from build123d import *

# Parameters (mm, degrees)
SKICA1_R                 = 60
VYSUNOUT1_DEPTH          = 10
SKICA7_R                 = 7.5
ODEBRAT_VYSUNUT_M1_DEPTH = 11
KRUHOV_POLE1_COUNT       = 6


with BuildPart() as part:
    # Skica1 → Vysunout1 (new body)
    with BuildSketch(Plane.XY):
        Circle(SKICA1_R)
    extrude(amount=VYSUNOUT1_DEPTH)

    # Skica7 → Odebrat vysunutím1 (cut, through all)
    with BuildSketch(Plane(origin=(0, 0, 0), x_dir=(-1, 0, 0), z_dir=(0, 0, -1))):
        with Locations((0, 40)):
            Circle(SKICA7_R)
    odebrat_vysunut_m1 = extrude(amount=-ODEBRAT_VYSUNUT_M1_DEPTH, mode=Mode.SUBTRACT)

    # Kruhové pole1: Odebrat vysunutím1 ×6 about axis
    kruhov_pole1_axis = Axis((0, 0, 0), (0, 0, 1))
    for i in range(1, KRUHOV_POLE1_COUNT):
        add(odebrat_vysunut_m1.rotate(kruhov_pole1_axis, i * 360 / KRUHOV_POLE1_COUNT), mode=Mode.SUBTRACT)


solid = part.part
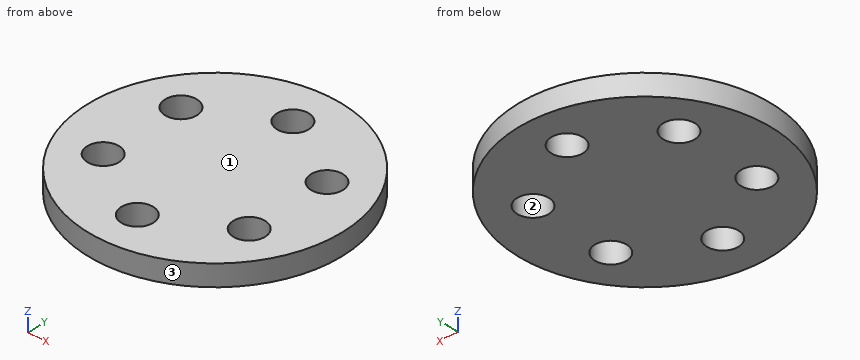
Part model, mm, in its own coordinate system. Face numbers are marked on the shaded views. Give positions to 0.01 mm unless a question says otherwise; leave off trailing zeros. Loops run counter-clockwise (first coordinate to the right, second up) from the corner with the lowest first, then second, coordinate; pieces in that order, holes last.
(1) Band-saw the part on D-D (y = 40). Write the cut outline in (x, z), and give its area (3 significant figures).
Return value:
outline: (-44.72, 0) - (-7.5, 0) - (-7.5, 10) - (-44.72, 10) - close; (7.5, 0) - (44.72, 0) - (44.72, 10) - (7.5, 10) - close
area: 744 mm2
(2) Drill centre lines: line 1 along Y through (x, z) = (-0.5, 2.5); line 2 along X through (y, z) = (18, 8.5); line 3 along Y through (x, z) = (41, 4.25). Where is each one in solid material? Low to high.
Return value:
line 1: y = -60 to -47.48, -32.52 to 32.52, 47.48 to 60
line 2: x = -57.24 to -41.87, -27.41 to 27.41, 41.87 to 57.24
line 3: y = -43.81 to -23.98, -16.02 to 16.02, 23.98 to 43.81
(3) Band-saw the part on A-A (x = 0). Write the cut outline in (y, z).
Return value:
outline: (-60, 0) - (-47.5, 0) - (-47.5, 10) - (-60, 10) - close; (-32.5, 0) - (32.5, 0) - (32.5, 10) - (-32.5, 10) - close; (47.5, 0) - (60, 0) - (60, 10) - (47.5, 10) - close
(4) Band-saw the part on B-B (y = -18.5). Write the cut outline in (x, z), and give its area (3 significant figures).
Return value:
outline: (-57.08, 0) - (-41.99, 0) - (-41.99, 10) - (-57.08, 10) - close; (-27.29, 0) - (27.29, 0) - (27.29, 10) - (-27.29, 10) - close; (41.99, 0) - (57.08, 0) - (57.08, 10) - (41.99, 10) - close
area: 848 mm2
(5) Pin check, flat tips, straight feed: pin 1 (5 mm diameter, centred on y = -26, z = 8, fed in from +X); pin 2 (1 mm diameter, centred on x = -37, z = 4, fed in from -Y); pin 3 (1.5 mm diameter, centred on x = -22, z = 1.5, fed in from -Y); pin 4 (9 mm diameter, centred on x = -34.64, y = 20, fed in from +Z). Stop position of each tip, or through.
Return value:
pin 1: stops at x = 55.21
pin 2: stops at y = -47.62
pin 3: stops at y = -56.11
pin 4: passes through
(6) Pull direction Y, two halves, no side cores. Call the marked faces 1, 2 and 3: pulls with the +Y half, pulls with the -Y half, needs draft (parallel to the pull), parting line crosses it, or undercut.
Return value:
face 1: needs draft
face 2: undercut
face 3: parting line crosses it
(7) Band-saw the part on C-C (z = 8). Write the cut outline in (x, y).
Return value:
outline: circle Ø120 at (0, 0); hole circle Ø15 at (-34.64, -20); hole circle Ø15 at (-34.64, 20); hole circle Ø15 at (0, -40); hole circle Ø15 at (0, 40); hole circle Ø15 at (34.64, -20); hole circle Ø15 at (34.64, 20)
